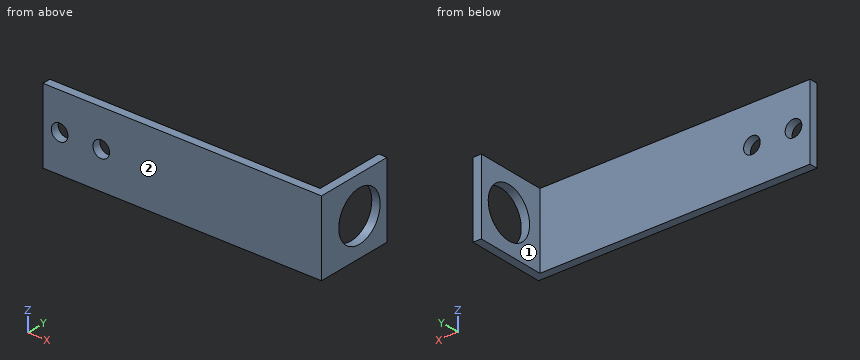
from build123d import *

# Parameters (mm, degrees)
BOSS_EXTRUDE1_DEPTH = 18
CUT_EXTRUDE1_REACH  = 4
SKETCH2_R           = 6
CUT_EXTRUDE2_REACH  = 4
SKETCH3_R           = 2


with BuildPart() as part:
    # Sketch1 → Boss-Extrude1 (new body)
    with BuildSketch(Plane.XY):
        Polygon((0, 0), (0, 19), (-2, 19), (-2, 2), (-67, 2), (-67, 0), align=None)
    extrude(amount=BOSS_EXTRUDE1_DEPTH)

    # Sketch2 → Cut-Extrude1 (cut, up to next)
    with BuildSketch(Plane.ZY.offset(2), mode=Mode.PRIVATE) as cut_extrude1_sk1:
        with Locations((9, 11)):
            Circle(SKETCH2_R)
    cut_extrude1_tool1 = extrude(cut_extrude1_sk1.sketch, amount=-CUT_EXTRUDE1_REACH, mode=Mode.PRIVATE) & part.part
    add(cut_extrude1_tool1.solids().sort_by_distance((-2, 11, 9))[0], mode=Mode.SUBTRACT)

    # Sketch3 → Cut-Extrude2 (cut, up to next)
    with BuildSketch(Plane(origin=(0, 2, 0), x_dir=(1, 0, 0), z_dir=(0, 1, 0)), mode=Mode.PRIVATE) as cut_extrude2_sk1:
        with Locations((-63, -9)):
            Circle(SKETCH3_R)
    cut_extrude2_tool1 = extrude(cut_extrude2_sk1.sketch, amount=-CUT_EXTRUDE2_REACH, mode=Mode.PRIVATE) & part.part
    add(cut_extrude2_tool1.solids().sort_by_distance((-63, 2, 9))[0], mode=Mode.SUBTRACT)
    # Sketch3 → Cut-Extrude2 (cut, up to next)
    with BuildSketch(Plane(origin=(0, 2, 0), x_dir=(1, 0, 0), z_dir=(0, 1, 0)), mode=Mode.PRIVATE) as cut_extrude2_sk2:
        with Locations((-53, -9)):
            Circle(SKETCH3_R)
    cut_extrude2_tool2 = extrude(cut_extrude2_sk2.sketch, amount=-CUT_EXTRUDE2_REACH, mode=Mode.PRIVATE) & part.part
    add(cut_extrude2_tool2.solids().sort_by_distance((-53, 2, 9))[0], mode=Mode.SUBTRACT)


solid = part.part
Source: CAD feature listing. Evaluate the final solid. Frame: model axes, mm. Face numbers are marked on the shaded views. A direction names the side the tool comes from. Round coordinates to 2 decimals unless told otherwise and drop trailing zeros. Loops run counter-clockwise (first coordinate to the right, second up) from the corner with the lowest first, then second, coordinate; pieces in that order, holes last. Notation, with made-up numbers: (31, -15) - (45, -15) arc R13 cw to (45, -4) - close; hole circle Ø4 at (-18.75, 53.25). An arc over 180 degrees is marked (long way). Write item = value, one per line. Start each with the question number.
(1) Ray query, line 1 along X through (y, z) = (1.4, 9); line 2 along Y through (x, z) = (-0.65, 9); line 3 along Y through (x, z) = (-3.5, 14). Return the intervals inside material, ascending. Write a range as from..to.
(2) Section query C-C, the plane y = 11. Output: boundary loops of the cut face in (x, z), plus the area to 3 significant figures.
(3) Section query B-B, the plane x = -63. Output: boundary loops of the cut face in (y, z), plus the area to 3 significant figures.
(4) Section query A-A, the plane z = 9. Output: boundary loops of the cut face in (x, y).
(5) Section query D-D, the plane z = 11.75. Output: boundary loops of the cut face in (x, y), plus the area to 3 significant figures.
(6) Pin query (flat end, axial travel): pin 1 (8 mm diameter, centred on x = -28, z = 14.5, fed in from -Y); pin 2 (3.5 mm diameter, centred on x = -63, z = 9, fed in from +Y); pin 3 (10 mm diameter, centred on y = 12, z = 12.5, fed in from -X); pin 4 (5 mm diameter, centred on x = -28.5, z = 12.5, fed in from +Y). Return the tip coordinate at first contact, or that it passes through.
(7) Set-up query: the marked faces 1 and 2. Return all of +Z, -Z, +X, -X, +Y, -Y with unobstructed straight access to the full face (end or side cutting, diameter ignored); none if empty.
Conclusion:
q1.line_1 = -67..-65, -61..-55, -51..0
q1.line_2 = 0..5, 17..19
q1.line_3 = 0..2
q2.outline = (-2, 0) - (0, 0) - (0, 3) - (-2, 3) - close; (-2, 15) - (0, 15) - (0, 18) - (-2, 18) - close
q2.area = 12.0 mm2
q3.outline = (0, 0) - (2, 0) - (2, 7) - (0, 7) - close; (0, 11) - (2, 11) - (2, 18) - (0, 18) - close
q3.area = 28.0 mm2
q4.outline = (-67, 0) - (-65, 0) - (-65, 2) - (-67, 2) - close; (-61, 0) - (-55, 0) - (-55, 2) - (-61, 2) - close; (-51, 0) - (0, 0) - (0, 5) - (-2, 5) - (-2, 2) - (-51, 2) - close; (-2, 17) - (0, 17) - (0, 19) - (-2, 19) - close
q5.outline = (-67, 0) - (0, 0) - (0, 5.67) - (-2, 5.67) - (-2, 2) - (-67, 2) - close; (-2, 16.33) - (0, 16.33) - (0, 19) - (-2, 19) - close
q5.area = 147 mm2
q6.pin_1 = 0
q6.pin_2 = through
q6.pin_3 = -2
q6.pin_4 = 2
q7.face_1 = +Z, -Z, -X, +Y
q7.face_2 = +Z, -Z, +X, -X, -Y
